```python
from build123d import *

# Parameters (mm, degrees)
SKETCH1_R           = 3.775
SKETCH1_R_2         = 2.2
BOSS_EXTRUDE1_DEPTH = 35
BOSS_EXTRUDE2_START = -6
SKETCH2_R           = 7.5
SKETCH2_R_2         = 3.775
BOSS_EXTRUDE2_DEPTH = 6
SKETCH3_W           = 6
SKETCH3_H           = 2
CUT_EXTRUDE1_DEPTH  = 37.571847096
SKETCH4_R           = 1.5
CUT_EXTRUDE2_DEPTH  = 37.571847096


with BuildPart() as part:
    # Sketch1 → Boss-Extrude1 (new body)
    with BuildSketch(Plane.XY):
        Circle(SKETCH1_R)
        Circle(SKETCH1_R_2, mode=Mode.SUBTRACT)
    extrude(amount=BOSS_EXTRUDE1_DEPTH)

    # Sketch2 → Boss-Extrude2 (add)
    with BuildSketch(Plane.XY.offset(35).offset(BOSS_EXTRUDE2_START)):
        Circle(SKETCH2_R)
        Circle(SKETCH2_R_2, mode=Mode.SUBTRACT)
    extrude(amount=BOSS_EXTRUDE2_DEPTH)

    # Sketch3 → Cut-Extrude1 (cut, through all)
    with BuildSketch(Plane.XY.offset(35)):
        with Locations((0, 4.5)):
            Rectangle(SKETCH3_W, SKETCH3_H)
        with Locations((0, -4.5)):
            Rectangle(SKETCH3_W, SKETCH3_H)
    extrude(amount=-CUT_EXTRUDE1_DEPTH, mode=Mode.SUBTRACT)

    # Sketch4 → Cut-Extrude2 (cut, through all)
    with BuildSketch(Plane(origin=(0, 0, 0), x_dir=(1, 0, 0), z_dir=(0, 1, 0))):
        with Locations(Location((0, -32, 0), (0, 0, 270))):
            Circle(SKETCH4_R)
    extrude(amount=-CUT_EXTRUDE2_DEPTH, mode=Mode.SUBTRACT)


solid = part.part
```
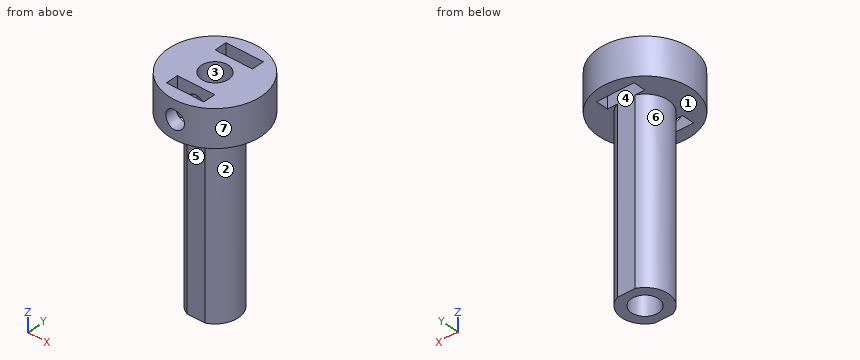
Geometry: final body of the model. Coordinates: model frame, mm. Face numbers are marked on the shaded views. A direction names the side the tool comes from. Round coordinates to 2 decimals unless told otherwise and drop trailing zeros. Order: outer loops, then holes, each group sorted by start corner. A loop starts at its lowest first (then second) coordinate and runs counter-clockwise, first axis right, second up. Notation, with made-up numbers: (49.25, -22) - (104.25, -22) arc R12 ccw to (104.25, -9) - close; hole circle Ø3 at (-34, 75). An arc over 180 degrees is marked (long way). Write item = value, one per line. Start each with the question number.
Q1. Cut plane C-C on z = 22.5. Return the cut outline in (x, y) (3 decimals), and give its area (3 significant figures).
Q2. Cut plane A-A on x = 0. Return the cut outline in (y, z).
Q3. Pull-direction query (X, two-part tool) for the marked faces 4, 5, 6 and 7; classes: +X half, -X half, draft (parallel to the pull), parting line (faces both ways), or undercut.
Q4. Ray query, line 1 (Z direction, x = 0, y = -6.45); line 2 (Y direction, x = 0, z = 11); line 3 (Z direction, x = 0, y = -2.4). Return the intervals inside material, ascending. Write a range as from..to.
Q5. Cut plane B-B on y = -6. Return the cut outline in (x, z).
Q6. Pin query (flat end, axial travel): pin 1 (5 mm diameter, centred on x = 1, z = 10, fed in from +Y); pin 2 (1.5 mm diameter, centred on y = -4, z = 4, fed in from -X); pin 3 (1.8 mm diameter, centred on x = 1.5, z = 31, fed in from +Y). Return the tip coordinate at first contact, or that it passes through.
Q7. Access query for the marked faces 1, 2 and 3. Directions: +Z, -Z, +X, -X, +Y, -Y. A direction counts if a zero-diameter tool reaches every point of the face in a straight line with its end or side. Return the directions, or none.
Q8. Cut plane D-D on x = 6. Return the cut outline in (y, z), and give its area (3 significant figures).
Outcome:
q1.outline = (-1.414, -3.5) - (1.414, -3.5) arc R3.775 ccw to (1.414, 3.5) - (-1.414, 3.5) arc R3.775 ccw to start; hole circle Ø4.4 at (0, 0)
q1.area = 28.5 mm^2
q2.outline = (-7.5, 29) - (-5.5, 29) - (-5.5, 30.5) - (-7.5, 30.5) - close; (-7.5, 33.5) - (-5.5, 33.5) - (-5.5, 35) - (-7.5, 35) - close; (-3.5, 0) - (-2.2, 0) - (-2.2, 30.5) - (-3.5, 30.5) - close; (-3.5, 33.5) - (-2.2, 33.5) - (-2.2, 35) - (-3.5, 35) - close; (2.2, 0) - (3.5, 0) - (3.5, 35) - (2.2, 35) - close; (5.5, 29) - (7.5, 29) - (7.5, 35) - (5.5, 35) - close
q3.face_4 = undercut
q3.face_5 = undercut
q3.face_6 = -X half
q3.face_7 = parting line
q4.line_1 = 29..30.5, 33.5..35
q4.line_2 = -3.5..-2.2, 2.2..3.5
q4.line_3 = 0..30.5, 33.5..35
q5.outline = (-4.5, 29) - (4.5, 29) - (4.5, 35) - (-4.5, 35) - close; hole circle Ø3 at (0, 32)
q6.pin_1 = 3.5
q6.pin_2 = -1.92
q6.pin_3 = 7.48
q7.face_1 = -Z
q7.face_2 = -Z, +X
q7.face_3 = +Z, -Z
q8.outline = (-4.5, 29) - (4.5, 29) - (4.5, 35) - (-4.5, 35) - close
q8.area = 54.0 mm^2
